Could you check a few things on this model? Use its own coordinates, in mm. Give positions to 0.01 mm unless a question says otherwise; leave off trailing zeros. Order: outer loops, then holes, each group sorted by start corner. A loop starts at its lowest first (then second) coordinate and runs counter-clockwise, first axis right, second up.
(1) Imagine slicing it at B-B, the plane y = 23.5. Write out the boundary of the cut face in (x, z).
(2) Will these pins go through, and if not, where does the flat tip stop? pin 1 (1.5 mm diameter, centred on x = -13.5, y = 41, fed in from -Z); pin 2 (6 mm diameter, centred on x = 39.5, y = 13.5, fed in from -Z); pin 3 (4 mm diameter, centred on x = -24.5, y = 16.5, fed in from +Z); pin 4 (7.5 mm diameter, centred on x = 0, z = 0, fed in from -Y).
(3) If we mould it in two halves opening along X, with no side actions, what happens to faces 1 (the cylindrical face through (4.877, 24.363, 0.215)), 2 (the flat face through (45, 0, -19))? For each: released by +X, released by -X, zero draft, split by the parting line, or undercut.
(4) Imagine slicing it at C-C, the plane x = -42.5. Write out the boundary of the cut face in (y, z), then the cut area to 3 significant figures.
(5) If I drill on probe 1 along Z at (x, y) = (0, 17); probe 2 along Z at (x, y) = (0, 24); probe 3 along Z at (x, y) = (-21, 28), over which ranges is the centre line in solid material (lowest first)?
(6) Imagine slicing it at D-D, the plane z = -20.5. Write out the boundary of the cut face in (x, y), then the cut area to 3 significant figures.
(7) Imagine slicing it at A-A, the plane x = 0. Write out the boundary of the cut face in (y, z).
from build123d import *

# Parameters (mm, degrees)
F1_ANGLE = 180
F2_D     = 4.7625
F4_T     = -2.5


# Not quite as in the source:
# - a feature of the source that left no trace in its solid (it failed there, or was rolled back) is left out


with BuildPart() as f1:
    # F0 (on Front) → F1 (revolve)
    with BuildSketch(Plane.XZ):
        with BuildLine():
            ThreePointArc((0, -50.8), (35.9210244843, -35.9210244843), (50.8, 0))
            ThreePointArc((50.8, 0), (35.9210244843, 35.9210244843), (0, 50.8))
            Line((0, 50.8), (0, 0))
            Line((0, 0), (0, -50.8))
        make_face()
    revolve(axis=Axis((0, 0, 25.4), (0, 0, 1)), revolution_arc=F1_ANGLE)

    # F2 (through all)
    with Locations(Plane.XZ):
        with Locations((0, 0)):
            Hole(F2_D / 2)

    # F4
    f4_openings = [f1.faces().sort_by_distance(p)[0] for p in [
        (49.363159, 0, 0),
    ]]
    offset(amount=F4_T, openings=f4_openings)


solid = f1.part
Answer block:
1. outline: circle Ø90.08 at (0, 0); circle Ø9.76 at (0, 0); hole circle Ø84.4 at (0, 0); hole circle Ø4.76 at (0, 0)
2. pin 1: stops at z = -27.96
2. pin 2: stops at z = -32.86
2. pin 3: stops at z = 42.69
2. pin 4: stops at y = 0
3. face 1: undercut
3. face 2: zero draft
4. outline: (0, -27.83) arc R27.83 ccw to (0, 27.83) - (0, 22.95) arc R22.95 cw to (0, -22.95) - close
4. area: 389 mm2
5. probe 1: z = -47.87 to -45.21, -4.88 to -2.38, 2.38 to 4.88, 45.21 to 47.87
5. probe 2: z = -44.77 to -41.92, -4.88 to -2.38, 2.38 to 4.88, 41.92 to 44.77
5. probe 3: z = -36.82 to -33.28, 33.28 to 36.82
6. outline: (-46.48, 0) - (-43.73, 0) arc R43.73 cw to (43.73, 0) - (46.48, 0) arc R46.48 ccw to start
6. area: 389 mm2
7. outline: (0, -50.8) arc R50.8 ccw to (50.74, -2.38) - (0, -2.38) - (0, -4.88) - (48.05, -4.88) arc R48.3 cw to (0, -48.3) - close; (0, 2.38) - (50.74, 2.38) arc R50.8 ccw to (0, 50.8) - (0, 48.3) arc R48.3 cw to (48.05, 4.88) - (0, 4.88) - close
